Geometry: final body of the model. Coordinates: model frame, mm. Give positions to 0.01 mm unless a question says otherwise; leave off trailing zeros. Loops run counter-clockwise (first coordinate to the right, second up) from the corner with the lowest first, then second, coordinate; pieces in that order, holes last.
```python
from build123d import *

# Parameters (mm, degrees)
F1_DEPTH  = 1.6
F2_R      = 3
F3_DEPTH  = 3
F6_R      = 0.5
F7_R      = 0.5
F8_R      = 0.5
F5_R      = 0.425
F4_R      = 0.5
F9_DEPTH  = 4
F10_R     = 2.1
F11_DEPTH = 0.2


with BuildPart() as f1:
    # F0 (on Top) → F1 (new body)
    with BuildSketch(Plane.XY):
        with BuildLine():
            Line((70.716411, 29.285482), (6.37358, 29.285482))
            ThreePointArc((6.37358, 29.285482), (38.544995, 6.285482), (70.716411, 29.285482))
        make_face()
    extrude(amount=F1_DEPTH)

    # F2 (on face) → F3 (cut)
    with BuildSketch(Plane.XY.offset(1.6)):
        with Locations((14.544995, 23.785482)):
            Circle(F2_R)
        with Locations((62.544995, 23.785482)):
            Circle(F2_R)
    extrude(amount=-F3_DEPTH, mode=Mode.SUBTRACT)

    # F6 (on face) + F7 (on face) + F8 (on face) + F5 (on face) + F4 (on face) → F9 (cut)
    with BuildSketch(Plane.XY.offset(1.6)):
        with Locations((48.844995, 14.685482)):
            Circle(F6_R)
        with Locations((53.844995, 14.685482)):
            Circle(F6_R)
        with Locations((51.344995, 14.685482)):
            Circle(F6_R)
    with BuildSketch(Plane.XY.offset(1.6)):
        with Locations((37.294995, 26.285482)):
            Circle(F7_R)
        with Locations((39.794995, 26.285482)):
            Circle(F7_R)
    with BuildSketch(Plane.XY.offset(1.6)):
        with Locations((36.794995, 14.585482)):
            Circle(F8_R)
        with Locations((40.294995, 14.585482)):
            Circle(F8_R)
    with BuildSketch(Plane.XY.offset(1.6)):
        with BuildLine():
            ThreePointArc((50.394995, 21.135482), (50.144995, 20.885482), (50.394995, 20.635482))
            Line((50.394995, 20.635482), (52.294995, 20.635482))
            ThreePointArc((52.294995, 20.635482), (52.544995, 20.885482), (52.294995, 21.135482))
            Line((52.294995, 21.135482), (50.394995, 21.135482))
        make_face()
        with Locations((48.164995, 22.585482)):
            Circle(F5_R)
        with Locations((54.524995, 22.585482)):
            Circle(F5_R)
    with BuildSketch(Plane.XY.offset(1.6)):
        with Locations((23.544995, 21.285482)):
            Circle(F4_R)
        with Locations((25.544995, 21.285482)):
            Circle(F4_R)
        with Locations((27.544995, 21.285482)):
            Circle(F4_R)
    extrude(amount=-F9_DEPTH, mode=Mode.SUBTRACT)

    # F10 (on face) → F11 (cut)
    with BuildSketch(Plane(origin=(0, 0, 0), x_dir=(1, 0, 0), z_dir=(0, 0, -1))):
        with Locations((62.544995, -23.785482)):
            Circle(F10_R)
        with Locations((14.544995, -23.785482)):
            Circle(F10_R)
    extrude(amount=-F11_DEPTH, mode=Mode.SUBTRACT)


solid = f1.part
```
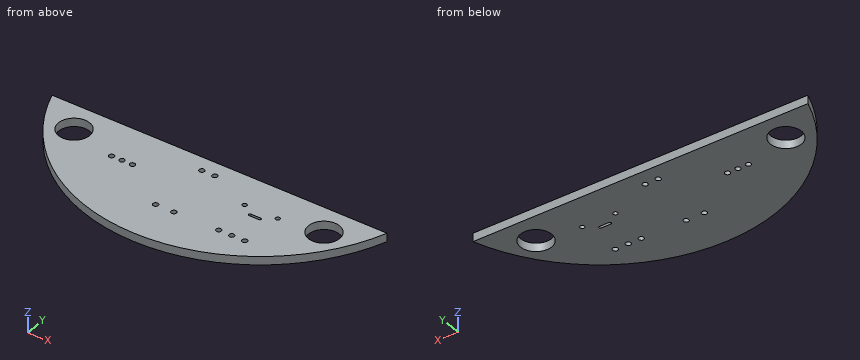
Q1. Section query B-B, the plane z = 1.15. State how many separate pieces and enclosed holes the cut face has, and give its area (3 significant figures).
Q2. Section query C-C, the plane y = 16. Return loops of the section in (x, z), and give its area (3 significant figures).
Q3. Material intervals for probe 1 along Y at (x, z) = (51.5, 0.55); probe 2 along Y at (x, z) = (62, 1); probe 3 along Y at (x, z) = (41, 1.5), sorted ascending.
Q4. Section query A-A, the plane x = 62.5. Return loops of the section in (y, z).
Q5. Section query D-D, the plane y = 11.5. Return loops of the section in (x, z), and give its area (3 significant figures).
Resolved:
1. separate pieces: 1
1. enclosed holes: 15
1. area: 1,010 mm2
2. outline: (14.75, 0) - (62.34, 0) - (62.34, 1.6) - (14.75, 1.6) - close
2. area: 76.1 mm2
3. probe 1: y = 8.85 to 14.21, 15.16 to 20.64, 21.14 to 29.29
3. probe 2: y = 15.67 to 20.84, 26.74 to 29.29
3. probe 3: y = 6.37 to 29.29
4. outline: (16.16, 0) - (20.79, 0) - (20.79, 1.6) - (16.16, 1.6) - close; (26.79, 0) - (29.29, 0) - (29.29, 1.6) - (26.79, 1.6) - close
5. outline: (20.45, 0) - (56.64, 0) - (56.64, 1.6) - (20.45, 1.6) - close
5. area: 57.9 mm2
